Geometry: see drawing. Coordinates: mm, zero at the bounding-box minimum. Give positions to 0.01 mm unless a question says otherwise; leave off trailing zeros. Write each loop counter-clockwise with the first axis right and the second up, starting at its lowest first coordinate (ties: lowest second). Pieces come first, ordered by that corner, then holes. Notation, with made-up numbers: (26.5, -26.5) - (61.5, -26.5) arc R14 ccw to (61.5, -22.5) - close; hole circle Ø10 at (-25, 53). An arc over 180 degrees is marked (long way). Use a Markdown table: item, result. Add a question column.
1. Section query A-A, the plane y = 38. Return loops of the section in (x, z), plus the area to 3 significant figures.
2. Section query B-B, the plane x = 4.85. Count the separate pieces of the cut face and the enclosed holes in it, plus the area to 3 significant figures.
3. Material intervals for probe 1 along Z at (x, y) = (5.3, 135); probe 2 along Y at (x, z) = (1.85, 54.5), sorted ascending.
4. Pin query (flat end, axial travel): pin 1 (1.8 mm diameter, centred on x = 4.5, z = 346, fed in from +Y); pin 2 (3 mm diameter, centred on x = 4.5, z = 71, fed in from +Y). Return the tip coordinate at first contact, or that it passes through.
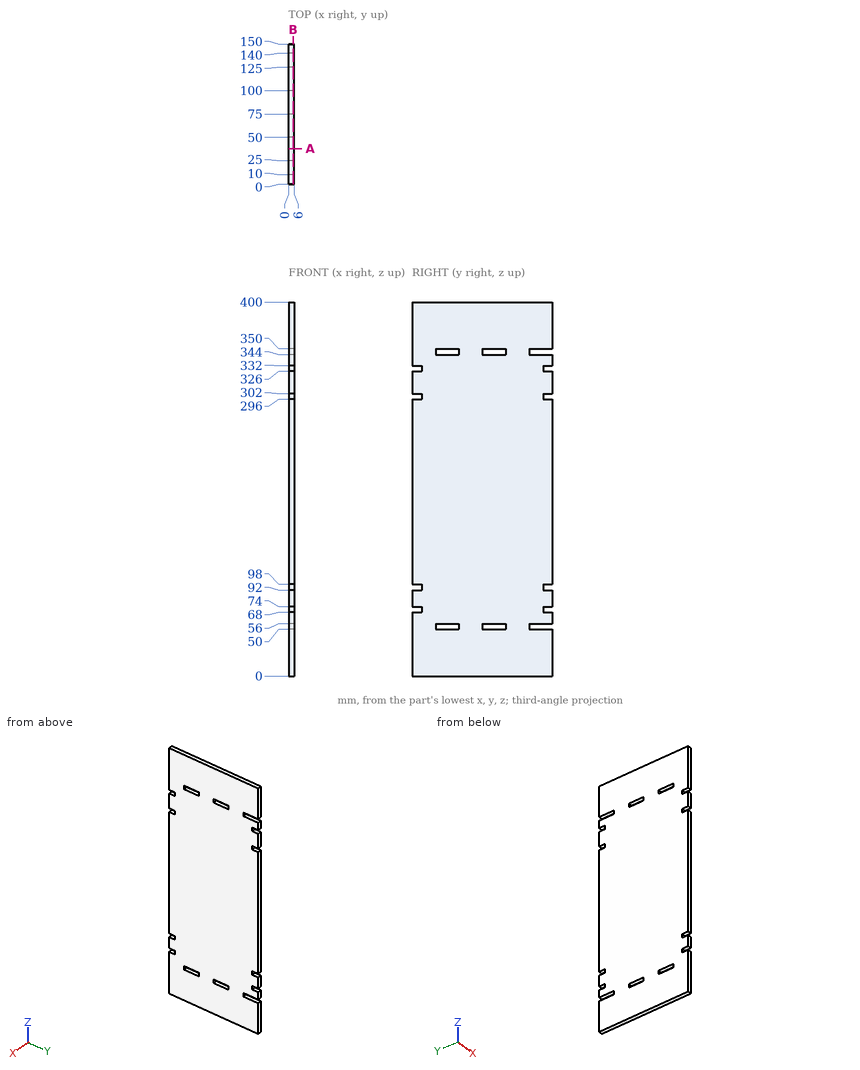
Result sheet:
| question | item | result |
|---|---|---|
| 1 | outline | (0, 0) - (6, 0) - (6, 50) - (0, 50) - close; (0, 56) - (6, 56) - (6, 344) - (0, 344) - close; (0, 350) - (6, 350) - (6, 400) - (0, 400) - close |
| 1 | area | 2,330 mm² |
| 2 | separate pieces | 1 |
| 2 | enclosed holes | 4 |
| 2 | area | 58,600 mm² |
| 3 | probe 1 | z = 0 to 50, 56 to 344, 350 to 400 |
| 3 | probe 2 | y = 0 to 25, 50 to 75, 100 to 125 |
| 4 | pin 1 | stops at y = 125 |
| 4 | pin 2 | stops at y = 140 |
